from build123d import *

# Parameters (mm, degrees)
F0_R     = 37.06963
F0_R_2   = 11.25
F1_DEPTH = 7
F2_R     = 2


with BuildPart() as f1:
    # F0 (on Top) → F1 (new body)
    with BuildSketch(Plane.XY):
        with Locations((-44.385914, -7.321505)):
            Circle(F0_R)
        with BuildLine():
            ThreePointArc((-17.383998, 8.268058), (-14.26919, 0.748247), (-13.206787, -7.321505))
            ThreePointArc((-13.206787, -7.321505), (-14.26919, -15.391257), (-17.383998, -22.911069))
            ThreePointArc((-17.383998, -22.911069), (-28.79635, -34.323421), (-44.385914, -38.500632))
            ThreePointArc((-44.385914, -38.500632), (-59.975477, -34.323421), (-71.38783, -22.911069))
            ThreePointArc((-71.38783, -22.911069), (-75.565041, -7.321505), (-71.38783, 8.268058))
            ThreePointArc((-71.38783, 8.268058), (-59.975477, 19.680411), (-44.385914, 23.857622))
            ThreePointArc((-44.385914, 23.857622), (-28.79635, 19.680411), (-17.383998, 8.268058))
        make_face(mode=Mode.SUBTRACT)
        with BuildLine():
            ThreePointArc((-30.778047, -7.321505), (-31.241724, -3.79953), (-32.601156, -0.517572))
            ThreePointArc((-32.601156, -0.517572), (-37.581981, 4.463253), (-44.385914, 6.286361))
            ThreePointArc((-44.385914, 6.286361), (-51.189847, 4.463253), (-56.170672, -0.517572))
            ThreePointArc((-56.170672, -0.517572), (-57.99378, -7.321505), (-56.170672, -14.125438))
            ThreePointArc((-56.170672, -14.125438), (-51.189847, -19.106263), (-44.385914, -20.929372))
            ThreePointArc((-44.385914, -20.929372), (-37.581981, -19.106263), (-32.601156, -14.125438))
            ThreePointArc((-32.601156, -14.125438), (-31.241724, -10.84348), (-30.778047, -7.321505))
        make_face()
        with Locations((-44.385914, -7.321505)):
            Circle(F0_R_2, mode=Mode.SUBTRACT)
        with BuildLine():
            ThreePointArc((-71.38783, -22.911069), (-59.975477, -34.323421), (-44.385914, -38.500632))
            Line((-44.385914, -38.500632), (-44.385914, -20.929372))
            ThreePointArc((-44.385914, -20.929372), (-51.189847, -19.106263), (-56.170672, -14.125438))
            Line((-56.170672, -14.125438), (-71.38783, -22.911069))
        make_face()
        with BuildLine():
            Line((-44.385914, 6.286361), (-44.385914, 23.857622))
            ThreePointArc((-44.385914, 23.857622), (-59.975477, 19.680411), (-71.38783, 8.268058))
            Line((-71.38783, 8.268058), (-56.170672, -0.517572))
            ThreePointArc((-56.170672, -0.517572), (-51.189847, 4.463253), (-44.385914, 6.286361))
        make_face()
        with BuildLine():
            ThreePointArc((-17.383998, -22.911069), (-14.26919, -15.391257), (-13.206787, -7.321505))
            ThreePointArc((-13.206787, -7.321505), (-14.26919, 0.748247), (-17.383998, 8.268058))
            Line((-17.383998, 8.268058), (-32.601156, -0.517572))
            ThreePointArc((-32.601156, -0.517572), (-31.241724, -3.79953), (-30.778047, -7.321505))
            ThreePointArc((-30.778047, -7.321505), (-31.241724, -10.84348), (-32.601156, -14.125438))
            Line((-32.601156, -14.125438), (-17.383998, -22.911069))
        make_face()
    extrude(amount=F1_DEPTH)

    # F2
    f2_edges = [f1.edges().sort_by_distance(p)[0] for p in [
        (-81.455544, -7.321505, 0),
        (-81.455544, -7.321505, 7),
    ]]
    fillet(f2_edges, radius=F2_R)


solid = f1.part
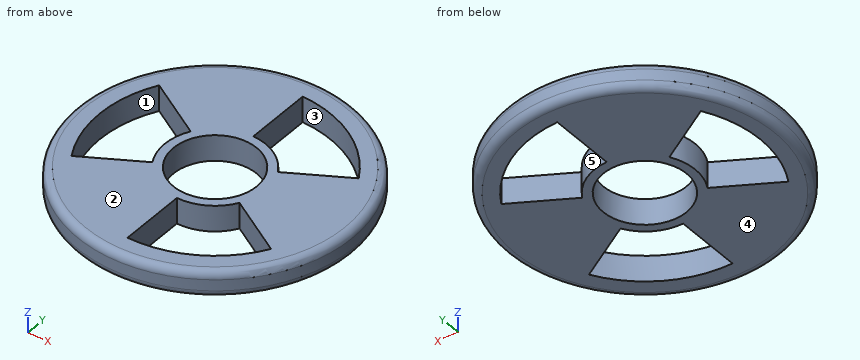
Input: part model. Units: mm. Frame: model coordinates. Face numbers are marked on the shaded views. A direction names the side the tool comes from. Give positions to 0.01 mm unless a question says otherwise; leave off trailing zeros. Loops run counter-clockwise (first coordinate to the right, second up) from the corner with the lowest first, then second, coordinate; pieces in that order, holes last. Notation, with made-up numbers: (-8, -10) -> (39, -10) arc R23 ccw to (39, 23) -> close; hole circle Ø10 at (50, 27.5). An arc over 180 degrees is marked (long way). Answer as a JSON object with one key per item and string values. Group by question number.
Item 1: Cut plane A-A, the plane z = 3.5. Return the cut outline in (x, y).
Item 2: Reachability of the marked faces 1 and 2 from +Z, -Z, +X, -X, +Y, -Y: full face, straight path, thin tool, end or side. Return the list, or none.
Item 3: Cut plane B-B, the plane y = -12. State how many separate pieces and enclosed holes the cut face has, and give its area (3 significant figures).
Item 4: Pin query (flat end, axial travel): P1, Ø4, axis at y = -12, z = 3.5, coming from the -X side; P2, Ø1.5, axis at y = 21.5, z = 1.5, coming from the +X side. Return the tip coordinate at first contact, or that it passes through.
Item 5: Pull-direction query (X, two-part tool) for the marked faces 3, 4 and 5; classes: released by +X, released by -X, zero draft, split by the parting line, or undercut.
Item 6: Line query: probe 1 along Y at (x, z) = (-44.5, 4.75); probe 2 along Y at (x, z) = (-37, 3.25); probe 3 along Y at (x, z) = (-30, 3.25). Output: solid intervals per line, ascending.
Checks:
{
 "1": {"outline": "circle Ø74.14 at (-44.39, -7.32); hole (-71.39, -22.91) -> (-56.17, -14.13) arc R13.61 cw to (-56.17, -0.52) -> (-71.39, 8.27) arc R31.18 ccw to start; hole circle Ø22.5 at (-44.39, -7.32); hole (-44.39, -38.5) arc R31.18 ccw to (-17.38, -22.91) -> (-32.6, -14.13) arc R13.61 cw to (-44.39, -20.93) -> close; hole (-44.39, 6.29) arc R13.61 cw to (-32.6, -0.52) -> (-17.38, 8.27) arc R31.18 ccw to (-44.39, 23.86) -> close"},
 "2": {"face 1": "+Z, -Z", "face 2": "+Z, +X, -X, +Y, -Y"},
 "3": {"separate pieces": "3", "enclosed holes": "0", "area": "242 mm²"},
 "4": {"P1": "stops at x = -81.36", "P2": "stops at x = -20.24"},
 "5": {"face 3": "undercut", "face 4": "zero draft", "face 5": "undercut"},
 "6": {"probe 1": "y = -44.39 to -18.57, 3.93 to 29.75", "probe 2": "y = -43.65 to -37.61, -18.75 to -15.81, 1.16 to 4.11, 22.97 to 29", "probe 3": "y = -41.49 to -34.98, -15.63 to 0.98, 20.34 to 26.84"}
}
